from build123d import *

# Parameters (mm, degrees)
SKETCH1_W           = 450
SKETCH1_H           = 170
BOSS_EXTRUDE1_DEPTH = 30
CHAMFER1_SIZE       = 11.88755803
CHAMFER1_SIZE_2     = 170
SKETCH2_R           = 4
BOSS_EXTRUDE2_DEPTH = 15
SKETCH3_W           = 280
SKETCH3_H           = 97
SKETCH3_W_2         = 20
SKETCH3_H_2         = 18
SKETCH3_W_3         = 77
SKETCH3_W_4         = 58.5
SKETCH3_H_3         = 38
BOSS_EXTRUDE3_DEPTH = 7.5


with BuildPart() as part:
    # Sketch1 → Boss-Extrude1 (new body)
    with BuildSketch(Plane(origin=(0, 0, 0), x_dir=(1, 0, 0), z_dir=(0, 1, 0))):
        with Locations((225, 85)):
            Rectangle(SKETCH1_W, SKETCH1_H)
    extrude(amount=BOSS_EXTRUDE1_DEPTH)

    # Chamfer1
    # the kernel refuses this chamfer: 170, 11.88755803 mm, written as the material it takes off along each edge
    with BuildSketch(Plane(origin=(-441.960179797, 30, 0), x_dir=(0, -0.8766829747338916, 0.48106856248536445), z_dir=(1, 0, 0))) as chamfer1_piece_1:
        Polygon((CHAMFER1_SIZE * 0.876682974763, CHAMFER1_SIZE * 0.481068562501), (-CHAMFER1_SIZE_2 * 0.481068562485, CHAMFER1_SIZE_2 * 0.876682974734), (0, 0), align=None)
    extrude(amount=1333.920359594, mode=Mode.SUBTRACT)

    # Sketch2 → Boss-Extrude2 (add)
    with BuildSketch(Plane(origin=(0, 0, -170), x_dir=(-1, 0, 0), z_dir=(0, 0, -1))):
        with Locations(Location((-105, 15, 0), (0, 0, 180))):
            Circle(SKETCH2_R)
    extrude(amount=BOSS_EXTRUDE2_DEPTH)

    # Sketch3 → Boss-Extrude3 (add)
    with BuildSketch(Plane(origin=(0, 18.02430745, 1.260382357), x_dir=(1, 0, 0), z_dir=(0, 0.9975640502598245, 0.06975647374412289))):
        Polygon((296.5, 16.263460083), (356.5, 16.263460083), (356.5, 34.263460083), (336.5, 34.263460083), (336.5, 52.263460083), (316.5, 52.263460083), (316.5, 34.263460083), (296.5, 34.263460083), align=None)
        with Locations((149, 64.763460083)):
            Rectangle(SKETCH3_W, SKETCH3_H)
        with Locations((19, 136.678582756)):
            Rectangle(SKETCH3_W_2, SKETCH3_H_2)
        with Locations((72.5, 136.678582756)):
            Rectangle(SKETCH3_W_3, SKETCH3_H_2)
        with Locations((153.5, 136.678582756)):
            Rectangle(SKETCH3_W_3, SKETCH3_H_2)
        with Locations((234.5, 136.678582756)):
            Rectangle(SKETCH3_W_3, SKETCH3_H_2)
        with Locations((325.75, 136.678582756)):
            Rectangle(SKETCH3_W_4, SKETCH3_H_2)
        with Locations((325.75, 94.263460083)):
            Rectangle(SKETCH3_W_4, SKETCH3_H_3)
        with Locations((402.5, 64.763460083)):
            Rectangle(SKETCH3_W_3, SKETCH3_H)
    extrude(amount=BOSS_EXTRUDE3_DEPTH)


solid = part.part
Verification items for the finished model (mm, model axes). A direction names the side the tool comes from. Give positions to 0.01 mm unless a question says otherwise; leave off trailing zeros. Order: outer loops, then holes, each group sorted by start corner. A loop starts at its lowest first (then second) coordinate and runs counter-clockwise, first axis right, second up. Notation, with made-up numbers: M -25,41 L -10,41 A5 ccw -10,46 Z; hole C -12,76.5 d2. An arc over 180 degrees is marked long. Answer as a JSON object with one key per item and string values. Group by question number.
1) Cross-section at B-B (z = -59). Enter the section's corners in (x, y).
2) Scan lines: line 1 along X through (y, z) = (27, -49.5); line 2 along X through (y, z) = (25, -16.5); line 3 along Y through (x, z) = (391.5, -144). Record each from-to range of solid material in increasing order. Write a range as [from, to].
3) Access from +Z, -Z, +X, -X, +Y, -Y to the whole of each face (thin tool, end or side, straight path). Record for faces 1 (the face through (18.86, 30.62, -125.85)), 2 (the face through (326.08, 22.847, -14.706)), 3 (the face through (306.64, 24.1, -32.66)), 4 (the face through (325.34, 26.963, -73.562)).
4) Mould release check, pull along X, two halves, no side actions. Record for faces 5 (the face through (222, 15, -170)), 6 (the face through (29, 31, -135)), 7 (the face through (102.05, 12.3, -177.4)): released by +X, released by -X, zero draft, split by the parting line, or undercut.
5) Cross-section at D-D (x = 105). Enter the section's corners in (y, z), then the cut area to 3 significant figures.
6) Depth check by flat-ended pin: pin 1 Ø11 at (y, z) = (26, -94.5) entering from +X; pin 2 Ø2.5 at (y, z) = (29.5, -133) entering from +X; pin 3 Ø7 at (y, z) = (26.5, -67.5) entering from -X; pin 4 Ø3 at (x, y) = (383, 26) entering from +Z. Enter the tip coordinate at first touch or a pass-through.
7) Cross-section at C-C (y = 4.5). Enter the section's corners in (x, z), then the cut area to 3 significant figures.
8) Cross-section at A-A (x = 256). Enter the section's corners in (y, z), then the cut area to 3 significant figures.
Result sheet:
{
 "1": {"outline": "M 0,0 L 450,0 L 450,22.24 L 441,22.24 L 441,29.76 L 364,29.76 L 364,22.24 L 289,22.24 L 289,29.76 L 9,29.76 L 9,22.24 L 0,22.24 Z"},
 "2": {"line 1": "x = [9, 289], [316.5, 336.5], [364, 441]", "line 2": "x = [9, 289], [296.5, 356.5], [364, 441]", "line 3": "y = [0, 28.18]"},
 "3": {"face 1": "+X, -X", "face 2": "+Z, +X, -X", "face 3": "+Y", "face 4": "none"},
 "4": {"face 5": "zero draft", "face 6": "undercut", "face 7": "split by the parting line"},
 "5": {"outline": "M 0,-170 L 11,-170 L 11,-185 L 19,-185 L 19,-170 L 30,-170 L 28.19,-144.06 L 35.67,-143.54 L 34.41,-125.58 L 26.93,-126.11 L 25.93,-111.73 L 33.41,-111.2 L 26.64,-14.44 L 19.16,-14.96 L 18.11,0 L 0,0 Z", "area": "5,070 mm2"},
 "6": {"pin 1": "stops at x = 450", "pin 2": "stops at x = 355", "pin 3": "stops at x = 9", "pin 4": "stops at z = -14.44"},
 "7": {"outline": "M 0,-170 L 450,-170 L 450,0 L 0,0 Z", "area": "76,500 mm2"},
 "8": {"outline": "M 0,-170 L 30,-170 L 28.19,-144.06 L 35.67,-143.54 L 34.41,-125.58 L 26.93,-126.11 L 25.93,-111.73 L 33.41,-111.2 L 26.64,-14.44 L 19.16,-14.96 L 18.11,0 L 0,0 Z", "area": "4,950 mm2"}
}
